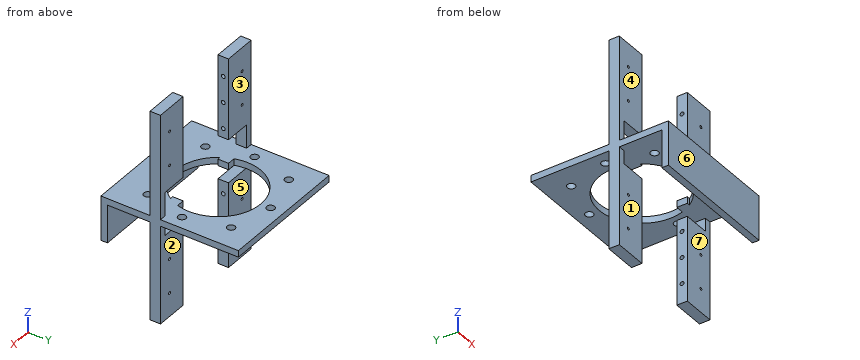
Autodesk Inventor part; units mm, degrees
ref_plane "Work Plane1" through (0, 0, 10.5) normal (0, 0, 1) x (1, 0, 0)
ref_plane "YZ Plane" through (0, 0, 0) normal (1, 0, 0) x (0, 1, 0)
ref_plane "XZ Plane" through (0, 0, 0) normal (0, 1, 0) x (-1, 0, 0)
sketch "Sketch1" plane through (0, 0, 0) normal (0, 0, 1) x (1, 0, 0)
  circle A0 centre (0, 0) radius 30 construction
  line L0 (0, 0) -> (0, 7.5) construction
  line L1 (0, 7.5) -> (10, 7.5) construction
  line L2 (10, 7.5) -> (10, 0) construction
  line L3 (10, 0) -> (0, 0) construction
  line L4 (0, 0) -> (-10, 0) construction
  line L5 (-10, 0) -> (-10, 7.5) construction
  line L6 (-10, 7.5) -> (0, 7.5) construction
  line L7 (-10, 0) -> (-10, -7.5) construction
  line L8 (-10, -7.5) -> (10, -7.5) construction
  line L9 (10, -7.5) -> (10, 0) construction
  circle A1 centre (-15.5891, 25.6316) radius 10 construction
  circle A2 centre (0, 0) radius 35 construction
  circle A3 centre (0, 0) radius 25 construction
  line L10 (0, 0) -> (-31.8198, 31.8198) construction
  circle A4 centre (0, 0) radius 45 construction
  line L11 (0, 0) -> (0, 45) construction
  circle A5 centre (0, 0) radius 40 construction
  circle A6 centre (-40, 0) radius 5 construction
  circle A7 centre (-31.8198, 31.8198) radius 10 construction
  line L12 (-31.8198, 31.8198) -> (-31.8198, -24.2384) construction
  line L13 (-31.8198, -24.2384) -> (-31.8198, -31.8198) construction
  circle A8 centre (-31.8198, -31.8198) radius 10 construction
  line L14 (-15, -20) -> (-15, -31.6228)
  line L15 (15, -20) -> (15, -31.6228)
  line L16 (-31.8198, 31.8198) -> (24.2384, 31.8198) construction
  line L17 (24.2384, 31.8198) -> (31.8198, 31.8198) construction
  line L18 (31.8198, 31.8198) -> (31.8198, -31.8198) construction
  line L19 (31.8198, -31.8198) -> (-31.8198, -31.8198) construction
  circle A9 centre (31.8198, 31.8198) radius 10 construction
  circle A10 centre (31.8198, -31.8198) radius 10 construction
  circle A11 centre (0, 40) radius 5 construction
  line L20 (0, 0) -> (40, 0) construction
  line L21 (0, 0) -> (0, -40) construction
  circle A12 centre (40, 0) radius 5 construction
  circle A13 centre (0, -40) radius 5 construction
  line L22 (50, 50) -> (50, -50)
  line L23 (50, -50) -> (-50, -50)
  line L24 (-50, -50) -> (-50, 50)
  line L25 (-50, 50) -> (50, 50)
  circle A14 centre (-31.8198, 31.8198) radius 3
  circle A15 centre (31.8198, 31.8198) radius 3
  circle A16 centre (31.8198, -31.8198) radius 3
  circle A17 centre (-31.8198, -31.8198) radius 3
  circle A18 centre (0, 0) radius 32.5
  point P0 (0, 50)
  dimension "d1" = 60
  dimension "d5" = 5
  dimension "d6" = 5
  dimension "d9" = 80
  dimension "d2" = 20
  dimension "d3" = 15
  dimension "d4" = 20
  dimension "d7" = 90
  dimension "d8" = 45
  dimension "d10" = 10
  dimension "d11" = 20
  dimension "d12" = 15
  dimension "d13" = 100
  dimension "d14" = 6
  dimension "d15" = 65
extrude "Extrusion1" add sketch "Sketch1" against normal blind 5
sketch "Sketch2" plane through (50, -50, 0) normal (1, 0, 0) x (0, 0, -1)
  line L0 (0, 0) -> (5, 0)
  line L1 (5, 0) -> (34, 0)
  line L2 (5, 0) -> (0, 0)
  line L3 (0, 0) -> (0, -5)
  line L4 (0, -5) -> (34, -5)
  line L5 (34, -5) -> (34, 0)
  dimension "d18" = 29
  dimension "d27" = 5
extrude "Extrusion2" add sketch "Sketch2" against normal up to surface (100 mm away)
ref_plane "Work Plane1" through (0, 0, 10.5) normal (0, 0, 1) x (1, 0, 0)
sketch "Sketch3" plane through (0, 0, 10.5) normal (0, 0, 1) x (1, 0, 0)
  line L0 (-8, -7.5) -> (8, -7.5)
  line L1 (10, -5.5) -> (10, 5.5)
  line L2 (8, 7.5) -> (-8, 7.5)
  line L3 (-10, 5.5) -> (-10, -5.5)
  arc A0 (-8, 7.5) -> (-10, 5.5) centre (-8, 5.5) ccw
  arc A1 (10, 5.5) -> (8, 7.5) centre (8, 5.5) ccw
  arc A2 (8, -7.5) -> (10, -5.5) centre (8, -5.5) ccw
  arc A3 (-10, -5.5) -> (-8, -7.5) centre (-8, -5.5) ccw
  point P0 (0, 0)
  point P1 (10, 7.5)
  point P2 (10, -7.5)
  point P3 (-10, 7.5)
  dimension "d22" = 20
  dimension "d23" = 15
  dimension "d24" = 7.5
  dimension "d25" = 10
  dimension "d26" = 2
sketch "Sketch4" plane through (0, 0, 0) normal (0, 0, 1) x (1, 0, 0)
  circle A0 centre (0, 0) radius 32.5
  line L0 (50, -55) -> (-50, -55)
  line L1 (0, 0) -> (-32.5, 0) construction
  line L2 (0, 0) -> (0, -7.5) construction
  line L3 (0, -7.5) -> (-10, -7.5) construction
  line L4 (-10, -7.5) -> (-55, -7.5) construction
  line L5 (-50, -9.5) -> (-25, -9.5)
  line L6 (-25, -9.5) -> (-25, -17.5)
  line L7 (-25, -17.5) -> (-50, -17.5)
  line L8 (-50, -17.5) -> (-50, -9.5)
  line L9 (-25, -13.5) -> (-50, -13.5) construction
  line L10 (-50, 50) -> (-50, -55)
  dimension "d28" = 7.5
  dimension "d29" = 10
  dimension "d30" = 6
  dimension "d31" = 8
  dimension "d32" = 25
  dimension "d44" = 0
extrude "Extrusion3" add sketch "Sketch4" along normal blind 80 contours L5 L6 L7 A0 | A0 L7 L8 L5 picked at (-26.286, -13.9829)
sketch "Sketch5" plane through (-25, -17.5, 0) normal (1, 0, 0) x (0, 0, -1)
  line L0 (-80, 8) -> (-80, 0)
  line L1 (0, 4) -> (-80, 4) construction
  circle A0 centre (-25, 4) radius 1.5
  circle A1 centre (-45, 4) radius 1.5
  circle A2 centre (-65, 4) radius 1.5
  circle A3 centre (-25, 4) radius 6 construction
  circle A4 centre (-45, 4) radius 6 construction
  circle A5 centre (-65, 4) radius 6 construction
  line L2 (0, 67.5) -> (0, -37.5)
  dimension "d36" = 3
  dimension "d38" = 12
  dimension "d39" = 20
  dimension "d40" = 20
  dimension "d43" = 25
extrude "Extrusion4" cut sketch "Sketch5" against normal blind 10
mirror "Mirror1" about plane through (0, 0, 0) normal (1, 0, 0) of "Extrusion3", "Extrusion4"
mirror "Mirror2" about plane through (0, 0, 0) normal (0, 0, 1) of "Extrusion3", "Extrusion4", "Mirror1"
sketch "Sketch6" plane through (-50, -9.5, -5) normal (0, 1, 0) x (1, 0, 0)
  line L0 (18.9195, 0) -> (0, 0) construction
  line L1 (100, 0) -> (81.0805, 0) construction
  line L2 (100, 0) -> (100, 75)
  line L3 (100, 75) -> (75, 75)
  line L4 (0, 0) -> (25, 0)
  line L5 (25, 0) -> (25, 10)
  line L6 (25, 10) -> (0, 10) construction
  line L7 (0, 10) -> (0, 0) construction
  line L8 (75, 0) -> (100, 0)
  line L9 (100, 0) -> (100, 10) construction
  line L10 (100, 10) -> (75, 10) construction
  line L11 (75, 10) -> (75, 0)
  line L12 (5, 10) -> (5, 0)
  line L13 (95, 10) -> (95, 0)
  line L14 (95, 0) -> (75, 0)
  line L15 (75, 0) -> (75, 10)
  line L16 (75, 10) -> (95, 10)
  line L17 (95, 10) -> (95, 0)
  line L18 (5, 0) -> (25, 0)
  line L19 (25, 0) -> (25, 10)
  line L20 (25, 10) -> (5, 10)
  line L21 (5, 10) -> (5, 0)
  line L22 (100, -85) -> (75, -85)
  line L23 (100, -5) -> (100, -85)
  line L24 (81.0805, -5) -> (100, -5)
  line L25 (81.0805, 0) -> (81.0805, -5)
  line L26 (75, 75) -> (75, -85)
  line L27 (25, -85) -> (25, 75)
  dimension "d45" = 10
  dimension "d46" = 10
  dimension "d49" = 5
  dimension "d50" = 5
  dimension "d56" = 0
  dimension "d57" = 0
extrude "Extrusion5" cut sketch "Sketch6" against normal blind 10 contours L8 L11 L16 L13 | L12 L20 L5 L4
sketch "Sketch7" plane through (-50, -9.5, 0) normal (0, 1, 0) x (1, 0, 0)
  line L0 (0, 0) -> (18.9195, 0)
  line L1 (5, 0) -> (95, 0)
  line L2 (95, 0) -> (95, -18)
  line L3 (95, -18) -> (5, -18)
  line L4 (5, -18) -> (5, 0)
  line L5 (75, 80) -> (75, -80)
  line L6 (100, 0) -> (100, -80)
  line L7 (5, 5) -> (5, 15)
  line L8 (95, 15) -> (95, 5)
  point P0 (25, -80)
  point P1 (15, 0)
  point P2 (85, 0)
  dimension "d55" = 18
  dimension "d58" = 0
  dimension "d59" = 0
extrude "Extrusion6" cut sketch "Sketch7" against normal blind 10
sketch "Sketch8" plane through (0, 0, 0) normal (0, 0, 1) x (1, 0, 0)
  line L0 (-31.0805, -9.5) -> (-25, -9.5)
  arc A0 (31.0805, -9.5) -> (-31.0805, -9.5) centre (0, 0) ccw
  circle A1 centre (0, 0) radius 40 construction
  line L1 (0, 0) -> (0, 40) construction
  circle A2 centre (0, 40) radius 3
  dimension "d61" = 80
  dimension "d60" = 6
extrude "Extrusion7" cut sketch "Sketch8" against normal blind 10
pattern_circular "Circular Pattern1" count 4 over 360 about axis through (0, 0, 0) along (0, 0, -1) of "Extrusion7"
sketch "Sketch9" plane through (-50, -9.5, 80) normal (0, 1, 0) x (1, 0, 0)
  line L0 (0, 80) -> (0, 0)
  line L1 (12.5, 31) -> (0, 31) construction
  circle A0 centre (10, 44) radius 1
  circle A1 centre (10, 18) radius 1
  line L2 (18.9195, 80) -> (18.9195, 85)
  line L3 (10, 44) -> (10, 18) construction
  dimension "d67" = 2
  dimension "d68" = 13
  dimension "d69" = 13
  dimension "d72" = 10
extrude "Extrusion8" cut sketch "Sketch9" against normal blind 10
mirror "Mirror3" about plane through (0, 0, 0) normal (1, 0, 0) of "Extrusion8"
mirror "Mirror4" about plane through (0, 0, 0) normal (0, 0, 1) of "Extrusion8", "Mirror3"
properties part number "Base"
Geometry check sheet. Reference: the model listing, model coordinates, mm. Face numbers are marked on the shaded views. A direction names the side the tool comes from. Give positions to 0.01 mm unless a question says otherwise; leave off trailing zeros. Loops run counter-clockwise (first coordinate to the right, second up) from the corner with the lowest first, then second, coordinate; pieces in that order, holes last. Notation, with made-up numbers: M 43,6.5 L 96,6.5 A12 cw 96,18.5 Z; hole C 17,19 d9. An arc over 180 degrees is marked long. Write item = value, one per line. Start each with the question number.
1. Go/stop test with flat-tipped pins: P1, Ø8, axis at x = -31.5, z = -26.5, coming from the +Y side; P2, Ø23, axis at x = -12, z = -24, coming from the +Y side; P3, Ø9.5, axis at x = 0, y = -40, coming from the -Z side. Record where each tip stops, or that it passes through.
2. Draft check along Y on the marked faces 5, 6 and 7. Enter one of: +Y half, -Y half, draft (parallel to the pull), parting line (faces both ways), or undercut.
3. Section check B-B, the plane z = -52. Enter the section's corners in (x, y), plus the area to 3 significant figures.
4. Tool access check on the marked faces 1, 2, 3 and 4. Record the directions out of +Z, -Z, +X, -X, +Y, -Y that give a thin tool (end or side, any length) a straight path to the whole face; none if there is none.
5. Thickness scan on probe 1 along X at (y, z) = (-12, 62); probe 2 along Y at (x, z) = (0, -2.65); probe 3 along Y at (x, z) = (-28, 65). Record the ranges inside material, lowest first.
6. Section check A-A, the plane y = 40. Enter the section's corners in (x, z).
7. Section check C-C, the plane x = -12.5. Enter the section's corners in (y, z), plus the area to 3 significant figures.
Values follow:
q1.P1 = -9.5
q1.P2 = -50
q1.P3 = -5
q2.face_5 = +Y half
q2.face_6 = -Y half
q2.face_7 = undercut
q3.outline = M -50,-17.5 L -25,-17.5 L -25,-9.5 L -50,-9.5 Z; M 25,-17.5 L 50,-17.5 L 50,-9.5 L 25,-9.5 Z
q3.area = 400 mm^2
q4.face_1 = -Z, +X, -X
q4.face_2 = -Z, +X, -X, +Y
q4.face_3 = +Z, +X, -X, +Y
q4.face_4 = +Z, +X, -X, -Y
q5.probe_1 = -50 to -41, -39 to -25, 25 to 39, 41 to 50
q5.probe_2 = -55 to -43, -37 to -32.5, 32.5 to 37, 43 to 50
q5.probe_3 = -17.5 to -15, -12 to -9.5
q6.outline = M -50,-5 L -3,-5 L -3,0 L -50,0 Z; M 3,-5 L 50,-5 L 50,0 L 3,0 Z
q7.outline = M -55,-34 L -50,-34 L -50,-5 L -30,-5 L -30,0 L -55,0 Z; M 30,-5 L 50,-5 L 50,0 L 30,0 Z
q7.area = 370 mm^2
